Could you check a few things on this model? Use its own coordinates, in mm. A direction names the side the tool comes from. Round coordinates to 2 decimals unless told otherwise and drop trailing zeros. Write each loop counter-clockwise with the first axis right and the second up, starting at its lowest first coordinate (ties: lowest second). Pieces come first, ordered by that corner, then holes.
Autodesk Inventor part; units mm, degrees
ref_plane "YZ Plane" through (0, 0, 0) normal (1, 0, 0) x (0, 1, 0)
ref_plane "XZ Plane" through (0, 0, 0) normal (0, 1, 0) x (-1, 0, 0)
ref_plane "XY Plane" through (0, 0, 0) normal (0, 0, 1) x (1, 0, 0)
sketch "Sketch1" plane through (0, 0, 0) normal (0, 1, 0) x (-1, 0, 0)
  circle A0 centre (0, 0) radius 35.2
  dimension "d0" = 70.4
extrude "Extrusion1" add sketch "Sketch1" along normal blind 8
sketch "Sketch2" plane through (0, 8, 0) normal (0, 1, 0) x (1, 0, 0)
  circle A0 centre (0, 0) radius 14
  dimension "d3" = 28
extrude "Extrusion2" add sketch "Sketch2" along normal blind 45
sketch "Sketch3" plane through (0, 0, 0) normal (0, 0, 1) x (1, 0, 0)
  circle A0 centre (0, 45.5) radius 7.5
  point P0 (0, 0)
extrude "Extrusion3" add sketch "Sketch3" along normal blind 25
sketch "Sketch4" plane through (0, 45.5, 25) normal (0, 0, 1) x (1, 0, 0)
  circle A0 centre (0, 0) radius 31.5
  point P0 (0, -45.5)
  dimension "d8" = 63
extrude "Extrusion4" add sketch "Sketch4" along normal blind 82
sketch "Sketch5" plane through (0, 45.5, 107) normal (0, 0, 1) x (1, 0, 0)
  line L0 (-21.5, 13) -> (21.5, 13)
  line L1 (21.5, 13) -> (21.5, -13)
  line L2 (21.5, -13) -> (-21.5, -13)
  line L3 (-21.5, -13) -> (-21.5, 13)
  line L4 (-21.5, 13) -> (21.5, -13) construction
  line L5 (21.5, 13) -> (-21.5, -13) construction
  line L6 (-10, -20) -> (10, -20)
  line L7 (10, -20) -> (10, -28)
  line L8 (10, -28) -> (-10, -28)
  line L9 (-10, -28) -> (-10, -20)
  line L10 (-10, -20) -> (10, -28) construction
  line L11 (10, -20) -> (-10, -28) construction
  point P0 (0, -45.5)
  point P1 (0, 0)
  point P2 (0, -24)
  dimension "d11" = 43
  dimension "d12" = 26
  dimension "d13" = 20
  dimension "d14" = 8
extrude "Extrusion5" cut sketch "Sketch5" against normal blind 2
sketch "Sketch6" plane through (0, 45.5, 105) normal (0, 0, 1) x (1, 0, 0)
  circle A0 centre (0, 0) radius 7.5
  circle A1 centre (-5, -24) radius 5
  circle A2 centre (5, -24) radius 5
  point P0 (0, -45.5)
  point P1 (0, -24)
  dimension "d17" = 15
  dimension "d18" = 10
  dimension "d19" = 10
extrude "Extrusion6" add sketch "Sketch6" along normal blind 1
sketch "Sketch8" plane through (0, 0, 0) normal (0, -1, 0) x (1, 0, 0)
  circle A0 centre (0, 0) radius 28 construction
  line L0 (0, 0) -> (50, 0) construction
  line L1 (0, 0) -> (-43.3013, -25) construction
  line L2 (0, 0) -> (50, 0) construction
  line L3 (0, 0) -> (0, 50)
  line L4 (0, 0) -> (50, 0) construction
  circle A1 centre (0, 28) radius 2.3
  circle A2 centre (-24.2487, -14) radius 2.3
  line L5 (0, 0) -> (43.3013, -25) construction
  line L6 (0, 0) -> (50, 0) construction
  circle A3 centre (24.2487, -14) radius 2.3
  dimension "d22" = 56
  dimension "d26" = 50
  dimension "d27" = 210
  dimension "d28" = 50
  dimension "d29" = 90
  dimension "d30" = 4.6
  dimension "d31" = 4.6
  dimension "d34" = 50
  dimension "d35" = 30
  dimension "d36" = 4.6
extrude "Extrusion7" cut sketch "Sketch8" against normal blind 8
properties part number "camera real"
Q1. Imagine slicing it at D-D, the plane z = 0. Write out the boundary of the cut face in (x, y).
Q2. Imagine slicing it at A-A, the plane z = 28. Write out the boundary of the cut face in (x, y).
Q3. I'm going to push flat-ended pins straight in: pin 1 Ø6 at (x, y) = (1, 22) entering from +Z; pin 2 Ø4 at (x, z) = (18.5, 34.5) entering from +Y; pin 3 Ø2 at (x, z) = (1, 105.5) entering from -Y. Where does each tip first touch, or does it pass through?
Q4. We'd pull the mould along Y, two halves only. Please class faces 1 (the flat face through (0, 18, 105)), 2 (the flat face through (0, 0, 0)), 3 (the cylindrical face through (1.06, 3.94, 25.96)): pulls with the +Y half, pulls with the -Y half, needs draft (parallel to the pull), parting line crosses it, or undercut.
Q5. If I drill on L1, parallel to Z at x = 0, y = 3.75; L2, parallel to Z at x = 19, y = 37; L3, parallel to Z at x = 30, y = 55, over which ranges is the centre line in solid material (lowest first)?
Q6. Imagine slicing it at C-C, the plane y = 23.5. Write out the boundary of the cut face in (x, z), then the cut area to 3 significant figures.
Q7. Imagine slicing it at B-B, the plane x = 16. Write out the boundary of the cut face in (y, z).
Q8. On a 3-axis mill with a long thin cutter (end or side, diameter ignored), from which of +Z, -Z, +X, -X, +Y, -Y can I reach the whole of each face in a straight line? I mean faces 4 (the flat face through (5, 22, 106)), 5 (the cylindrical face through (3.461, 52.154, 18.318)), 6 (the cylindrical face through (-33.575, 3.944, -10.573)). Say none if no direction works.
Results found:
1. outline: (-35.2, 0) - (35.2, 0) - (35.2, 8) - (14, 8) - (14, 53) - (-14, 53) - (-14, 8) - (-35.2, 8) - close
2. outline: circle Ø63 at (0, 45.5); (-21.33, 0) - (-2.3, 0) - (-2.3, 8) - (-21.33, 8) - close; (2.3, 0) - (21.33, 0) - (21.33, 8) - (2.3, 8) - close
3. pin 1: stops at z = 106
3. pin 2: stops at y = 72.33
3. pin 3: stops at y = 14
4. face 1: undercut
4. face 2: pulls with the -Y half
4. face 3: needs draft
5. L1: z = -35.2 to 25.7, 30.3 to 35.2
5. L2: z = 25 to 105
5. L3: z = 25 to 107
6. outline: (-22.54, 25) - (22.54, 25) - (22.54, 107) - (10, 107) - (10, 105) - (9.58, 105) - (9.58, 106) - (0.42, 106) - (0.42, 105) - (-0.42, 105) - (-0.42, 106) - (-9.58, 106) - (-9.58, 105) - (-10, 105) - (-10, 107) - (-22.54, 107) - close; circle Ø28 at (0, 0)
6. area: 4,290 mm2
7. outline: (0, -31.35) - (8, -31.35) - (8, 31.35) - (0, 31.35) - close; (18.37, 25) - (72.63, 25) - (72.63, 107) - (58.5, 107) - (58.5, 105) - (32.5, 105) - (32.5, 107) - (18.37, 107) - close
8. face 4: +Z
8. face 5: none
8. face 6: -Y
